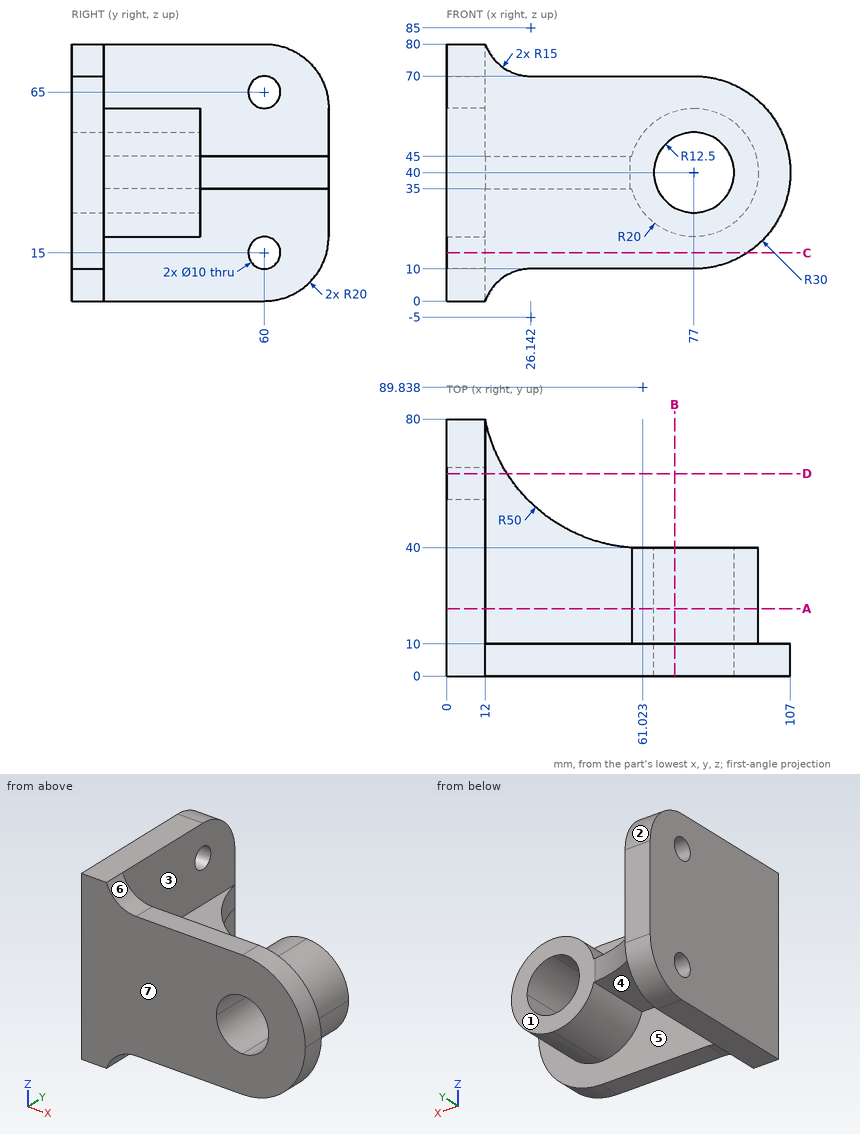
The drawing under review shows one solid part. Ordinate dimensions are in mm from its lowest x, y, z. A direction names the side the tool comes from. Coordinates: 2 decimals unless noted, no trailing zeros. Order: outer loops, then holes, each group sorted by start corner. A loop starts at its lowest first (then second) coordinate and runs counter-clockwise, first axis right, second up. Notation, with made-up numbers: (10, 66) -> (47, 66) arc R28 ccw to (47, 96) -> close; hole circle Ø11 at (38, 19.25). An arc over 180 degrees is marked (long way). Answer in a Markdown table with one row per item. Add a question column.
Item 1: To check wall thickness, follow probe 1 along X at (y, z) = (32, 34) (1 decimal); probe 2 along X at (y, z) = (31.5, 5); probe 3 along X at (y, z) = (6, 45.5) (1 decimal). State the ranges of each line that lie inside material, in increasing order.
Item 2: We need section C-C on z = 15. Write out the cut boundary in (x, y) (1 decimal).
Item 3: We need section A-A on y = 21. Write out the cut boundary in (x, z) (1 decimal).
Item 4: Clearance check with flat-ended pins moving along their axes: pin 1 (23 mm diameter, centred on x = 38, y = 34, fed in from -Z); pin 2 (2 mm diameter, centred on x = 94.5, y = 16.5, fed in from -Z); pin 3 (3 mm diameter, centred on x = 57.5, y = 6, fed in from -Z); pin 4 (9 mm diameter, centred on y = 60, z = 15, fed in from -X). State where each tip first meets the part, or that it passes through.
Item 5: We need section B-B on x = 71. Write out the cut boundary in (y, z).
Item 6: We need section D-D on y = 63. Write out the cut boundary in (x, z) (1 decimal).
Item 7: Mouldability with a two-part tool opening along X and no side actions: class the marked faces 4, 5, 6 and 7 as +X half, -X half, draft (parallel to the pull), parting line (faces both ways), or undercut.
Item 8: Machinability: for the marked faces 1, 2 and 3, which of the approach directions +Z, -Z, +X, -X, +Y, -Y give a long, thin tool a straight path to every point of the face, cutting with its end or side? Answer none if there is none.
Final values:
| question | item | result |
|---|---|---|
| 1 | probe 1 | x = 0 to 12, 57.9 to 66, 88 to 96.1 |
| 1 | probe 2 | x = 0 to 12 |
| 1 | probe 3 | x = 0 to 65.8, 88.2 to 106.5 |
| 2 | outline | (0, 0) -> (93.6, 0) -> (93.6, 10) -> (12, 10) -> (12, 55) -> (0, 55) -> close; (0, 65) -> (12, 65) -> (12, 79.4) -> (0, 79.4) -> close |
| 3 | outline | (0, 0) -> (12, 0) -> (12, 35) -> (57.6, 35) arc R20 ccw (long way) to (57.6, 45) -> (12, 45) -> (12, 80) -> (0, 80) -> close; hole circle Ø25 at (77, 40) |
| 4 | pin 1 | stops at z = 35 |
| 4 | pin 2 | stops at z = 28.7 |
| 4 | pin 3 | stops at z = 10 |
| 4 | pin 4 | passes through |
| 5 | outline | (0, 10) -> (10, 10) -> (10, 20.92) -> (40, 20.92) -> (40, 29.03) -> (0, 29.03) -> close; (0, 50.97) -> (40, 50.97) -> (40, 59.08) -> (10, 59.08) -> (10, 70) -> (0, 70) -> close |
| 6 | outline | (0, 0.2) -> (12, 0.2) -> (12, 11) -> (0, 11) -> close; (0, 19) -> (12, 19) -> (12, 35) -> (18.8, 35) -> (18.8, 45) -> (12, 45) -> (12, 61) -> (0, 61) -> close; (0, 69) -> (12, 69) -> (12, 79.8) -> (0, 79.8) -> close |
| 7 | face 4 | undercut |
| 7 | face 5 | undercut |
| 7 | face 6 | +X half |
| 7 | face 7 | draft |
| 8 | face 1 | +Z, -Z, +X, +Y |
| 8 | face 2 | +Z, +X, -X, +Y |
| 8 | face 3 | +Z, +Y |
